Work out the finished part from the listing and answer in its coordinate system (mm). Face numbers are marked on the shaded views. A direction names the side the tool comes from. Give positions to 0.01 mm unless a question says otherwise; leave off trailing zeros. Order: outer loops, then holes, each group sorted by start corner. A loop starts at its lowest first (then second) coordinate and runs counter-clockwise, first axis right, second up. Notation, with made-up numbers: (16, 18.25) - (23, 18.25) arc R25 cw to (23, 34.25) - close; hole circle Ø2 at (9.5, -18.5). An arc over 180 degrees is marked (long way). Put each result on its own line as item: value.
```python
from build123d import *

# Parameters (mm, degrees)
F0_R      = 10.9
F1_DEPTH  = 3
F2_R      = 9
F3_DEPTH  = 10
F4_R      = 13
F5_DEPTH  = 3
F7_DEPTH  = 7
F8_R      = 5
F9_DEPTH  = 9
F10_R     = 5
F11_DEPTH = 100
F13_R     = 15
F14_DEPTH = 25
F16_R     = 15
F17_DEPTH = 25
F18_R     = 5


with BuildPart() as f1:
    # F0 (on Top) → F1 (new body)
    with BuildSketch(Plane.XY):
        Circle(F0_R)
    extrude(amount=F1_DEPTH)

    # F2 (on face) → F3 (join)
    with BuildSketch(Plane.XY.offset(3)):
        Circle(F2_R)
    extrude(amount=F3_DEPTH)

    # F4 (on face) → F5 (join)
    with BuildSketch(Plane.XY.offset(13)):
        Circle(F4_R)
    extrude(amount=F5_DEPTH)

    # F6 (on face) → F7 (join)
    with BuildSketch(Plane.XY.offset(16)):
        Polygon((-5.484828, -9.5), (5.484828, -9.5), (10.969655, 0), (5.484828, 9.5), (-5.484828, 9.5), (-10.969655, 0), align=None)
    extrude(amount=F7_DEPTH)

    # F8 (on face) → F9 (join)
    with BuildSketch(Plane.XY.offset(23)):
        Circle(F8_R)
    extrude(amount=F9_DEPTH)

    # F10 (on face) → F11 (join)
    with BuildSketch(Plane(origin=(0, 0, 0), x_dir=(1, 0, 0), z_dir=(0, 0, -1))):
        Circle(F10_R)
    extrude(amount=F11_DEPTH)

    # F13 (on offset) → F14 (join)
    with BuildSketch(Plane(origin=(0, 0, -95), x_dir=(1, 0, 0), z_dir=(0, 0, -1))):
        Circle(F13_R)
    extrude(amount=-F14_DEPTH)

    # F16 (on offset) → F17 (join)
    with BuildSketch(Plane(origin=(0, 0, -35), x_dir=(1, 0, 0), z_dir=(0, 0, -1))):
        Circle(F16_R)
    extrude(amount=-F17_DEPTH)

    # F18
    f18_edges = [f1.edges().sort_by_distance(p)[0] for p in [
        (-15, 0, -70),
        (-15, 0, -95),
        (-15, 0, -10),
        (-15, 0, -35),
    ]]
    fillet(f18_edges, radius=F18_R)


solid = f1.part
```
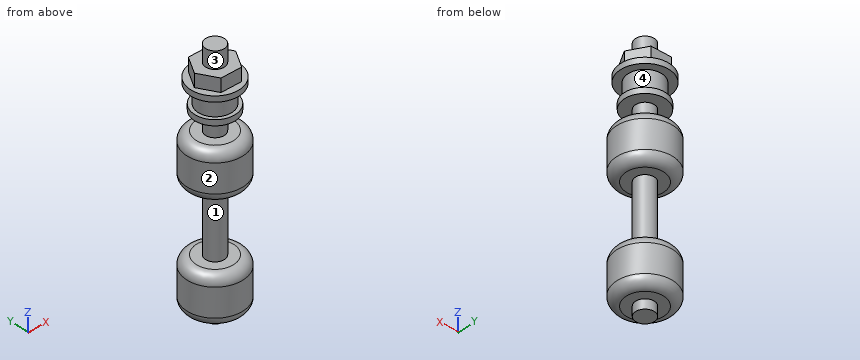
(1) Straight lines are drawn through the part: line 1 (Z direction, x = -7, y = 3); line 2 (Z direction, x = -9.5, y = 3.25); line 3 (Z direction, x = 6.5, y = -10.5). For each, find the intervals that lie inside material, in ascending order.
Geometry check:
line 1: z = -95 to -70, -35 to -10, 0 to 23
line 2: z = -95 to -70, -35 to -10, 0 to 3, 13 to 16
line 3: z = -94.41 to -70.59, -34.41 to -10.59, 13 to 16
(2) A tool of negligible diameter and unlimited length cuts with its end or side. For the marked faces 1 and 2, from which of +Z, -Z, +X, -X, +Y, -Y can it reach the whole face along a straight path? Write none if from no direction.
Geometry check:
face 1: none
face 2: +Z, -Z
(3) Determine the mould class of the marked faces 3 and 4 for opening direction Z: pulls with the +Z half, pulls with the -Z half, needs draft (parallel to the pull), parting line crosses it, or undercut.
Geometry check:
face 3: needs draft
face 4: undercut
(4) Given pin 1 (4 mm diameter, centred on x = 3, z = -75.5, fed in from -Y); pin 2 (2 mm diameter, centred on x = 0.5, z = 18, fed in from +Y); pin 3 (1.5 mm diameter, centred on x = -6.5, z = -50, fed in from +Y); pin 4 (7.5 mm diameter, centred on x = 0.5, z = 18, fed in from -Y), each flat-ended and moving along its own axis, determine where each tip first touches the part or whether it passes through.
Geometry check:
pin 1: stops at y = -14.97
pin 2: stops at y = 9.5
pin 3: passes through
pin 4: stops at y = -13
(5) Section A-A, the plane z = -22 is taken. Write down the section's boundary in (x, y), then the cut area to 3 significant figures.
Geometry check:
outline: circle Ø30 at (0, 0)
area: 707 mm²
